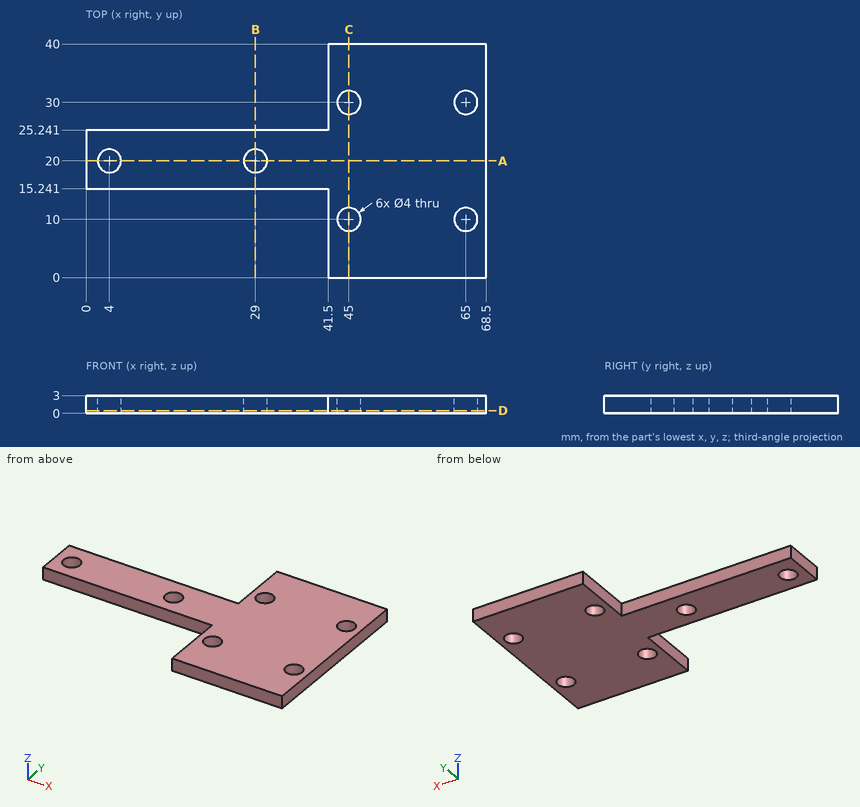
Drawing for the job (mm, zero at the part's lowest x, y, z). Round coordinates to 2 decimals unless told otherwise and drop trailing zeros. Loops run counter-clockwise (first coordinate to the right, second up) from the corner with the lowest first, then second, coordinate; pieces in that order, holes last.
1. Band-saw the part on B-B, the plane x = 29. List the corners of the cut face in (y, z).
Check values:
outline: (15.24, 0) - (18, 0) - (18, 3) - (15.24, 3) - close; (22, 0) - (25.24, 0) - (25.24, 3) - (22, 3) - close
2. Band-saw the part on C-C, the plane x = 45. List the corners of the cut face in (y, z).
Check values:
outline: (0, 0) - (8, 0) - (8, 3) - (0, 3) - close; (12, 0) - (28, 0) - (28, 3) - (12, 3) - close; (32, 0) - (40, 0) - (40, 3) - (32, 3) - close
3. Band-saw the part on A-A, the plane y = 20. List the corners of the cut face in (x, z).
Check values:
outline: (0, 0) - (2, 0) - (2, 3) - (0, 3) - close; (6, 0) - (27, 0) - (27, 3) - (6, 3) - close; (31, 0) - (68.5, 0) - (68.5, 3) - (31, 3) - close
4. Drop flat-ended pins along their axis: P1, Ø1.5, axis at x = 11.5, z = 1.5, coming from the +Y side; P2, Ø2.5, axis at x = 65, y = 30, coming from the +Z side; P3, Ø0.9, axis at y = 8.5, z = 1.5, coming from the -X side. Give the stop position or say it passes through.
Check values:
P1: stops at y = 25.24
P2: passes through
P3: stops at x = 41.5
5. Band-saw the part on D-D, the plane z = 0.45. List the corners of the cut face in (x, y), and give its area (3 significant figures).
Check values:
outline: (0, 15.24) - (41.5, 15.24) - (41.5, 0) - (68.5, 0) - (68.5, 40) - (41.5, 40) - (41.5, 25.24) - (0, 25.24) - close; hole circle Ø4 at (4, 20); hole circle Ø4 at (29, 20); hole circle Ø4 at (45, 10); hole circle Ø4 at (45, 30); hole circle Ø4 at (65, 10); hole circle Ø4 at (65, 30)
area: 1,420 mm2
6. Wall check: probe 1 along X at (y, z) = (20, 1.3); probe 2 along X at (y, z) = (10, 2.25); probe 3 along Y at (x, z) = (45, 1.65). Give the ranges that are in metal, low to high.
Check values:
probe 1: x = 0 to 2, 6 to 27, 31 to 68.5
probe 2: x = 41.5 to 43, 47 to 63, 67 to 68.5
probe 3: y = 0 to 8, 12 to 28, 32 to 40
